```python
from build123d import *

# Parameters (mm, degrees)
F0_R      = 2.06375
F1_DEPTH  = 12.7
F1_FACE_R = 2.06375
F5_R      = 2.5146
F6_DEPTH  = 0.254


with BuildPart() as f1:
    # F0 (on Front) → F1 (new body)
    with BuildSketch(Plane.XZ):
        Circle(F0_R)
    extrude(amount=F1_DEPTH)

    # F3: sweep along a path in F2
    with BuildLine(Plane.XY) as f3_path:
        Line((0, 0), (0, -19.05))
        Line((0, -19.05), (12.7, -19.05))
    # F1_face (on face) → F3 (sweep)
    with BuildSketch(Plane(origin=(0, 0, 0), x_dir=(1, 0, 0), z_dir=(0, 1, 0))):
        Circle(F1_FACE_R)
    sweep(path=f3_path.line, transition=Transition.RIGHT)

    # F4: sweep along a path in F2
    with BuildLine(Plane.XY) as f4_path:
        Line((0, 0), (0, -15.24))
        Line((0, -15.24), (12.115027858, -19.05))
    # F1_face (on face) → F4 (sweep)
    with BuildSketch(Plane(origin=(0, 0, 0), x_dir=(1, 0, 0), z_dir=(0, 1, 0))):
        Circle(F1_FACE_R)
    sweep(path=f4_path.line, transition=Transition.RIGHT)

    # F5 (on Front) → F6 (join)
    with BuildSketch(Plane.XZ):
        Circle(F5_R)
    extrude(amount=F6_DEPTH)


solid = f1.part
```
Can you work these out from the model? Positions are in its coordinate system, mm. A direction names the side the tool comes from. Round coordinates to 2 decimals unless told otherwise and drop trailing zeros. Loops run counter-clockwise (first coordinate to the right, second up) from the corner with the lowest first, then second, coordinate; pieces in that order, holes last. Notation, with made-up numbers: (50, -30) -> (101, -30) arc R27 ccw to (101, -8) -> close; hole circle Ø8 at (42, -35.75). An arc over 180 degrees is marked (long way). Answer in a Markdown table with one row per item.
Item 1: Suppose I cut it at C-C, the plane y = -2.5. List the corners of the cut face in (x, z) for me, plus the area to 3 significant figures.
Answer block:
| item | result |
|---|---|
| outline | circle Ø4.13 at (0, 0) |
| area | 13.4 mm² |
Item 2: Suppose I cut it at B-B, the plane x = -1.5. List the corners of the cut face in (y, z) for me, plus the area to 3 significant figures.
Answer block:
| item | result |
|---|---|
| outline | (-20.55, -1.42) -> (-0.25, -1.42) -> (-0.25, -2.02) -> (0, -2.02) -> (0, 2.02) -> (-0.25, 2.02) -> (-0.25, 1.42) -> (-20.55, 1.42) arc R2.06 ccw to start |
| area | 59.7 mm² |
Item 3: On a 3-axis mill with a long thin cutter (end or side, diameter ignored), from which of +Z, -Z, +X, -X, +Y, -Y can I reach the whole of each face in a straight line? I mean faces 1 (the flat face through (0, 0, 0)), 2 (the cylindrical face through (-2.06, -8.22, 0.09)). Say none if no direction works.
Answer block:
| item | result |
|---|---|
| face 1 | +Z, -Z, +X, -X, +Y |
| face 2 | none |
Item 4: Suppose I cut it at D-D, the plane z = -0.95. List the corners of the cut face in (x, y) for me.
Answer block:
| item | result |
|---|---|
| outline | (-2.33, -0.25) -> (-1.83, -0.25) -> (-1.83, -20.88) -> (12.7, -20.88) -> (12.7, -17.22) -> (12.4, -17.22) -> (1.83, -13.9) -> (1.83, -0.25) -> (2.33, -0.25) -> (2.33, 0) -> (-2.33, 0) -> close |
Item 5: Will these pins go through, and if not, where does the flat tip stop? P1, Ø1, axis at y = -17, z = 1, coming from the -X side; P2, Ø2, axis at x = 10, z = -0.5, coming from the +Y side; P3, Ø1.5, axis at x = 8, z = 2, coming from the +Y side.
Answer block:
| item | result |
|---|---|
| P1 | x = -2 |
| P2 | y = -15.93 |
| P3 | y = -15.99 |
Item 6: If I drill on probe 1 along Y at (x, z) = (-0.5, 2.3); probe 2 along X at (y, z) = (-3.5, -0.05); probe 3 along Y at (x, z) = (8, 0.6), over which ranges is the centre line in solid material (lowest first)?
Answer block:
| item | result |
|---|---|
| probe 1 | -0.25 to 0 |
| probe 2 | -2.06 to 2.06 |
| probe 3 | -21.02 to -15.69 |
Item 7: We'd pull the mould along X, two halves only. Please class faces 3 (the cylindrical face through (6.761, -15.204, -0.071)), 4 (the flat face through (12.7, -19, 0)), 5 (the flat face through (-2, -0.254, 1)): released by +X, released by -X, zero draft, split by the parting line, or undercut.
Answer block:
| item | result |
|---|---|
| face 3 | undercut |
| face 4 | released by +X |
| face 5 | zero draft |
